Design review of the part built by this model. Coordinates are the model's own, in mm. Give positions to 0.01 mm unless a question says otherwise; leave off trailing zeros. Write each loop counter-clockwise with the first axis right and the second up, starting at its lowest first coordinate (ties: lowest second). Pieces come first, ordered by that corner, then holes. Notation, with made-up numbers: (67, 0.25) -> (72, 0.25) arc R23 cw to (72, 10.25) -> close; hole circle Ø7 at (2.5, -13). An arc over 180 degrees is marked (long way). Answer as a JSON object with one key per item and string values.
```python
from build123d import *

# Parameters (mm, degrees)
F0_R     = 51.65308
F1_DEPTH = 50.8
F2_R     = 38.291887
F3_DEPTH = 50.038
F4_R     = 38.1


with BuildPart() as f1:
    # F0 (on Front) → F1 (new body)
    with BuildSketch(Plane.XZ):
        Circle(F0_R)
    extrude(amount=F1_DEPTH)

    # F2 (on face) → F3 (cut)
    with BuildSketch(Plane(origin=(0, 0, 0), x_dir=(-1, 0, 0), z_dir=(0, 1, 0))):
        Circle(F2_R)
    extrude(amount=-F3_DEPTH, mode=Mode.SUBTRACT)

    # F4
    f4_edges = [f1.edges().sort_by_distance(p)[0] for p in [
        (38.291887, -50.038, 0),
    ]]
    fillet(f4_edges, radius=F4_R)


solid = f1.part
```
(1) We need section B-B, the plane z = 45.5. State the section outline as (x, y) points, then the cut area to 3 significant figures.
Here are the results:
{"outline": "(-24.45, -50.8) -> (24.45, -50.8) -> (24.45, 0) -> (-24.45, 0) -> close", "area": "2,480 mm²"}
(2) For line 1 along Z through (x, y) = (0, -5); line 2 along Z through (x, y) = (-6.5, -26); line 3 along X through (y, z) = (-46.5, 5), list the stretches that pass through material, from the lowest coordinate up.
Here are the results:
{"line 1": "z = -51.65 to -38.29, 38.29 to 51.65", "line 2": "z = -51.24 to -35, 35 to 51.24", "line 3": "x = -51.41 to -15.44, 15.44 to 51.41"}
(3) We need section A-A, the plane x = 45. State the section outline as (y, z) points.
Here are the results:
{"outline": "(-50.8, -25.36) -> (0, -25.36) -> (0, 25.36) -> (-50.8, 25.36) -> close"}
(4) The part is to be moulded in two halves that separate along Z. For faces 1 (the cylindrical face through (30.387, -5.885, -23.3)), 2 (the cylindrical face through (49.268, -25.044, 15.515)), 3 (the flat face through (-1, -50.8, 1)), say which applies: +Z half, -Z half, draft (parallel to the pull), parting line (faces both ways), or undercut.
Here are the results:
{"face 1": "undercut", "face 2": "parting line", "face 3": "draft"}
(5) Clearance check with flat-ended pins moving along their axes: pin 1 (10 mm diameter, centred on x = 4.5, y = -18, fed in from -Z); pin 2 (3 mm diameter, centred on y = -39, z = 4, fed in from -X); pin 3 (4 mm diameter, centred on x = -35.5, y = -16, fed in from +Z). State where each tip first meets the part, or that it passes through.
Here are the results:
{"pin 1": "stops at z = -51.65", "pin 2": "stops at x = -51.59", "pin 3": "stops at z = 39.32"}
